from build123d import *

# Parameters (mm, degrees)
F4_R = 1


with BuildPart() as f1:
    # F0 (on Front) → F1 (revolve)
    with BuildSketch(Plane.XZ):
        Polygon((-30.1100046678, 10), (-25, 0), (-4, 0), (-4, 4), (-9.7, 4), (-9.7, 10), (-12.467299588, 10), (-12.467299588, 1), (-22.3023900814, 1), (-26.9013942824, 10), align=None)
    revolve(axis=Axis((0, 0, 12.4949840829), (0, 0, -1)))

    # F2 (on face) → F3 (join, up to the next surface of F1)
    with BuildSketch(Plane.XY.offset(10)):
        with BuildLine():
            ThreePointArc((1.5, 26.859542333), (0, 26.9013942824), (-1.5, 26.859542333))
            Line((-1.5, 26.859542333), (-1.5, 12.3767345862))
            ThreePointArc((-1.5, 12.3767345862), (0, 12.467299588), (1.5, 12.3767345862))
            Line((1.5, 12.3767345862), (1.5, 26.859542333))
        make_face()
        with BuildLine():
            Line((26.859542333, 1.5), (12.3767345862, 1.5))
            ThreePointArc((12.3767345862, 1.5), (12.467299588, 0), (12.3767345862, -1.5))
            Line((12.3767345862, -1.5), (26.859542333, -1.5))
            ThreePointArc((26.859542333, -1.5), (26.9013942824, 0), (26.859542333, 1.5))
        make_face()
        with BuildLine():
            Line((-12.3767345862, 1.5), (-26.859542333, 1.5))
            ThreePointArc((-26.859542333, 1.5), (-26.9013942824, 0), (-26.859542333, -1.5))
            Line((-26.859542333, -1.5), (-12.3767345862, -1.5))
            ThreePointArc((-12.3767345862, -1.5), (-12.467299588, 0), (-12.3767345862, 1.5))
        make_face()
        with BuildLine():
            ThreePointArc((1.5, -12.3767345862), (0, -12.467299588), (-1.5, -12.3767345862))
            Line((-1.5, -12.3767345862), (-1.5, -26.859542333))
            ThreePointArc((-1.5, -26.859542333), (0, -26.9013942824), (1.5, -26.859542333))
            Line((1.5, -26.859542333), (1.5, -12.3767345862))
        make_face()
    extrude(until=Until.NEXT, dir=(0, 0, -1))

    # F4
    f4_edges = [f1.edges().sort_by_distance(p)[0] for p in [
        (-1.5, 24.556037, 5.499836),
        (1.5, 24.556037, 5.499836),
        (-24.556037, 1.5, 5.499836),
        (-24.556037, -1.5, 5.499836),
        (-1.5, -24.556037, 5.499836),
        (24.556037, 1.5, 5.499836),
        (24.556037, -1.5, 5.499836),
        (1.5, -24.556037, 5.499836),
        (1.5, 12.376735, 5.5),
        (12.376735, 1.5, 5.5),
        (12.376735, -1.5, 5.5),
        (1.5, -12.376735, 5.5),
        (-1.5, -12.376735, 5.5),
        (-12.376735, -1.5, 5.5),
        (-12.376735, 1.5, 5.5),
        (-1.5, 12.376735, 5.5),
    ]]
    fillet(f4_edges, radius=F4_R)


solid = f1.part
Geometry check sheet. Reference: the model listing, model coordinates, mm. A direction names the side the tool comes from. Give positions to 0.01 mm unless a question says otherwise; leave off trailing zeros. Order: outer loops, then holes, each group sorted by start corner. A loop starts at its lowest first (then second) coordinate and runs counter-clockwise, first axis right, second up. Notation, with made-up numbers: M -7.75,-11 L 21.25,-11 A33 cw 21.25,22 Z; hole C 2,24 d5. An arc over 180 degrees is marked long. Use a Markdown table: item, result.
Item 1: Tool access check on faces 3 (the flat face through (0, -5, 0)), 4 (the flat face through (-1.5, 18, 6)). Record the directions out of +Z, -Z, +X, -X, +Y, -Y that give a thin tool (end or side, any length) a straight path to the whole face; none if there is none.
Answers follow:
| item | result |
|---|---|
| face 3 | -Z, +X, -X, +Y, -Y |
| face 4 | +Z |
Item 2: Draft check along X on faces 1 (the flat face through (12, -12, 1)), 2 (the flat face through (4.3, 9.1, 10)). Enter one of: +X half, -X half, draft (parallel to the pull), parting line (faces both ways), or undercut.
Answers follow:
| item | result |
|---|---|
| face 1 | undercut |
| face 2 | draft |
Item 3: Section check C-C (z = 3.25). State how many separate pieces and enclosed holes the cut face has, and give its area (3 significant figures).
Answers follow:
| item | result |
|---|---|
| separate pieces | 1 |
| enclosed holes | 5 |
| area | 1,080 mm2 |
Item 4: Section check A-A (y = 0). Record the cut outline in (x, z).
Answers follow:
| item | result |
|---|---|
| outline | M -30.11,10 L -25,0 L -4,0 L -4,4 L -9.7,4 L -9.7,10 Z; M 4,0 L 25,0 L 30.11,10 L 9.7,10 L 9.7,4 L 4,4 Z |
Item 5: Depth check by flat-ended pin: P1, Ø6, axis at x = 13.5, y = -11, coming from the +Z side; P2, Ø4, axis at x = 18, z = 5.5, coming from the -Y side; P3, Ø10, axis at x = -4.5, y = -10, coming from the -Z side; P4, Ø7, axis at x = 0, y = 0, coming from the -Z side. Enter the tip coordinate at first touch or a pass-through.
Answers follow:
| item | result |
|---|---|
| P1 | stops at z = 1 |
| P2 | stops at y = -23.22 |
| P3 | stops at z = 0 |
| P4 | passes through |
Item 6: Material ranges on line 1 along Y through (x, z) = (8, 7.5); line 2 along Y through (x, z) = (6, 2); line 3 along Y through (x, z) = (0, 1.3), recorded low to high.
Answers follow:
| item | result |
|---|---|
| line 1 | y = -27.7 to -24.34, -9.56 to -5.49, 5.49 to 9.56, 24.34 to 27.7 |
| line 2 | y = -25.32 to -22.01, -10.93 to 10.93, 22.01 to 25.32 |
| line 3 | y = -25.66 to -4, 4 to 25.66 |
